Geometry: final body of the model. Coordinates: model frame, mm. Give positions to 0.01 mm unless a question says otherwise; leave off trailing zeros. Order: outer loops, then holes, each group sorted by start corner. A loop starts at its lowest first (then second) coordinate and runs counter-clockwise, first axis right, second up. Notation, with made-up numbers: (-21.5, 51.5) - (-6.5, 51.5) arc R18 cw to (-6.5, 63.5) - close; hole circle Ø2 at (16, 71). An arc over 180 degrees is marked (long way). Put each result on its own line as item: value. Start each with the question number.
1. Ray query, line 1 along Y through (x, z) = (0.7, 15); line 2 along Z through (x, y) = (2.2, 148.5); line 3 along Z through (x, y) = (1, 132.75). Return the intervals inside material, ascending. Write a range as from..to.
2. Section B-B on y = 108. Return the cut outline in (x, z), plus the area to 3 significant figures.
3. Section A-A on y = 148.5. Return the cut outline in (x, z), plus the area to 3 significant figures.
4. Section C-C on x = 1.95. Count the separate pieces of the cut face and the enclosed holes in it, plus the area to 3 significant figures.
5. First-contact query: P1, Ø2, axis at x = 3.5, y = 40, coming from the +Z side; P2, Ø3, axis at y = 113.5, z = -4.25, coming from the +X side; P3, Ø4, axis at y = 132.75, z = 15, coming from the +X side; P4, Ø2, axis at x = 4.5, z = -1.5, coming from the +Y side. Flat tips, straight axial feed; report the tip coordinate or a pass-through.
6. Section D-D on z = 20.5. Return the cut outline in (x, y), plus the area to 3 significant figures.
from build123d import *

# Parameters (mm, degrees)
SKETCH_1_W                  = 5
SKETCH_1_H                  = 30
EXTRUDE_1_DEPTH             = 227
SKETCH_2_R                  = 22.5
EXTRUDE_2_DEPTH             = 5
SKETCH_3_R                  = 13
CUT_EXTRUDE_1_DEPTH         = 231.130940988
HOLE_WIZARD_M31_D           = 3.4
HOLE_WIZARD_M31_CBORE_D     = 6.7
HOLE_WIZARD_M31_CBORE_DEPTH = 2
HOLE_WIZARD_M41_D           = 4.5


with BuildPart() as part:
    # Эскиз1 → Бобышка-Вытянуть1 (new body)
    with BuildSketch(Plane(origin=(0, 0, 0), x_dir=(1, 0, 0), z_dir=(0, 1, 0))):
        with Locations((2.5, -15)):
            Rectangle(SKETCH_1_W, SKETCH_1_H)
    extrude(amount=EXTRUDE_1_DEPTH)

    # Эскиз2 → Бобышка-Вытянуть2 (add)
    with BuildSketch(Plane.ZY):
        with Locations((15, 113.5)):
            Circle(SKETCH_2_R)
    extrude(amount=-EXTRUDE_2_DEPTH)

    # Эскиз3 → Вырез-Вытянуть1 (cut, through all)
    with BuildSketch(Plane.ZY):
        with Locations((15, 113.5)):
            Circle(SKETCH_3_R)
    extrude(amount=-CUT_EXTRUDE_1_DEPTH, mode=Mode.SUBTRACT)

    # Цековка для  винта с полукруглой головкой M31 (through all)
    with Locations(Plane(origin=(5, -25.024735225, 7.262908886), x_dir=(0, 0, 1), z_dir=(1, 0, 0))):
        with Locations((7.737091114, -157.774735225), (-11.512908886, -138.524735225), (7.737091114, -119.274735225), (26.987091114, -138.524735225)):
            CounterBoreHole(HOLE_WIZARD_M31_D / 2, HOLE_WIZARD_M31_CBORE_D / 2, HOLE_WIZARD_M31_CBORE_DEPTH)

    # Отверстие с зазором M41 (through all)
    with Locations(Plane(origin=(5, 0, 0), x_dir=(0, 0, -1), z_dir=(1, 0, 0))):
        with Locations((-26, 148.5), (-4, 148.5), (-4, 78.5), (-26, 78.5)):
            Hole(HOLE_WIZARD_M41_D / 2)


solid = part.part
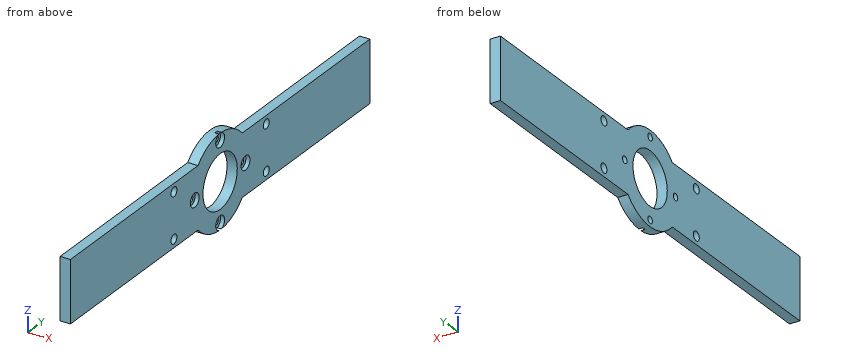
Resolved:
1. line 1: 0..92.55, 95.95..100.5, 126.5..131.05, 134.45..227
1. line 2: 0..1.75, 6.25..23.75, 28.25..30
1. line 3: 0..13.3, 16.7..30
2. outline: (0, -6.82) - (5, -6.82) - (5, 3.22) - (0, 3.22) - close; (0, 26.78) - (5, 26.78) - (5, 36.82) - (0, 36.82) - close
2. area: 100 mm^2
3. outline: (0, 0) - (5, 0) - (5, 1.75) - (0, 1.75) - close; (0, 6.25) - (5, 6.25) - (5, 23.75) - (0, 23.75) - close; (0, 28.25) - (5, 28.25) - (5, 30) - (0, 30) - close
3. area: 105 mm^2
4. separate pieces: 1
4. enclosed holes: 9
4. area: 6,530 mm^2
5. P1: z = 30
5. P2: through
5. P3: x = 3
5. P4: y = 129.81
6. outline: (0, 0) - (5, 0) - (5, 101.72) - (0, 101.72) - close; (0, 125.28) - (5, 125.28) - (5, 227) - (0, 227) - close
6. area: 1,020 mm^2
